Geometry: see drawing. Coordinates: mm, zero at the bounding-box minimum. A direction names the side the tool comes from. Coordinates: 2 decimals unless noted, no trailing zeros. Order: outer loops, then holes, each group sorted by start corner. A loop starts at its lowest first (then second) coordinate and runs counter-clockwise, first axis right, second up.
Item 1: Section A-A on z = 12.05. Return the cut outline in (x, y).
Item 2: Reachability of the marked faces 4 and 5 from +Z, -Z, +X, -X, +Y, -Y: full face, straight path, thin tool, end or side. Return the list, or none.
Item 3: Mould query, pull axis Y, two halves, no side actions, for the marked faces 1, 2 and 3. Classes: released by +Y, released by -Y, zero draft, split by the parting line, or undercut.
Item 4: Section B-B on x = 10. Return the cut outline in (y, z).
Item 5: Contact query for flat-ended pins moving along their axis: P1, Ø1, axis at x = 15.5, z = 6.5, coming from the +Y side; P2, Ø12, axis at x = 26.5, z = 19, coming from the +Y side (1 decimal). Output: stop coordinate, or through.
Item 6: Ray query, line 1 (X direction, y = 3.1, z = 12.05); line 2 (Z direction, x = 20, y = 22.5); line 3 (Y direction, x = 10, z = 1.3). Return the intervals inside material, ascending.
Item 7: Section C-C on y = 23. Return the cut outline in (x, z), then the cut area to 3 significant figures.
Item 8: Section D-D on x = 18. Return the cut outline in (y, z).
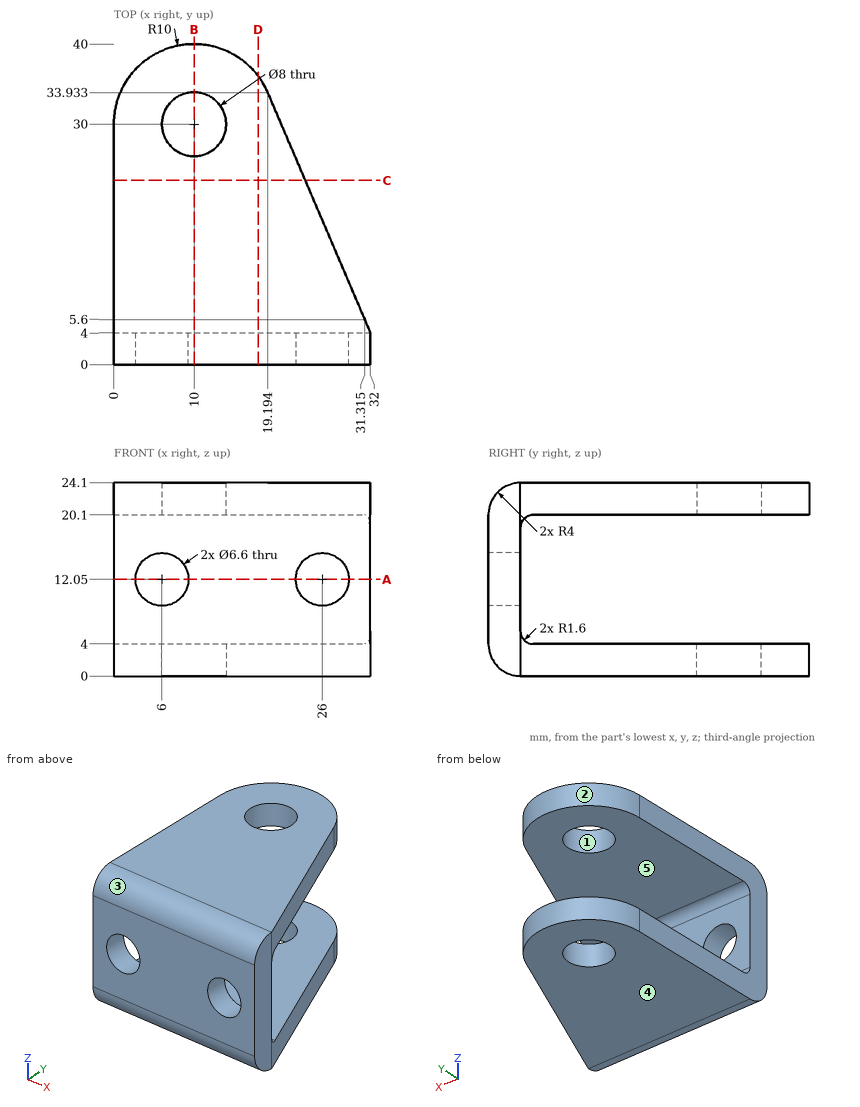
Answer list:
1. outline: (0, 0) - (2.7, 0) - (2.7, 4) - (0, 4) - close; (9.3, 0) - (22.7, 0) - (22.7, 4) - (9.3, 4) - close; (29.3, 0) - (32, 0) - (32, 4) - (29.3, 4) - close
2. face 4: -Z, +X, -X, +Y, -Y
2. face 5: +X, -X, +Y
3. face 1: undercut
3. face 2: released by +Y
3. face 3: released by -Y
4. outline: (0, 4) arc R4 ccw to (4, 0) - (26, 0) - (26, 4) - (5.6, 4) arc R1.6 cw to (4, 5.6) - (4, 18.5) arc R1.6 cw to (5.6, 20.1) - (26, 20.1) - (26, 24.1) - (4, 24.1) arc R4 ccw to (0, 20.1) - close; (34, 0) - (40, 0) - (40, 4) - (34, 4) - close; (34, 20.1) - (40, 20.1) - (40, 24.1) - (34, 24.1) - close
5. P1: stops at y = 4
5. P2: stops at y = 30.6
6. line 1: x = 0 to 2.7, 9.3 to 22.7, 29.3 to 32
6. line 2: z = 0 to 4, 20.1 to 24.1
6. line 3: y = 1.05 to 26, 34 to 40
7. outline: (0, 0) - (23.87, 0) - (23.87, 4) - (0, 4) - close; (0, 20.1) - (23.87, 20.1) - (23.87, 24.1) - (0, 24.1) - close
7. area: 191 mm2
8. outline: (0, 4) arc R4 ccw to (4, 0) - (36, 0) - (36, 4) - (5.6, 4) arc R1.6 cw to (4, 5.6) - (4, 18.5) arc R1.6 cw to (5.6, 20.1) - (36, 20.1) - (36, 24.1) - (4, 24.1) arc R4 ccw to (0, 20.1) - close
